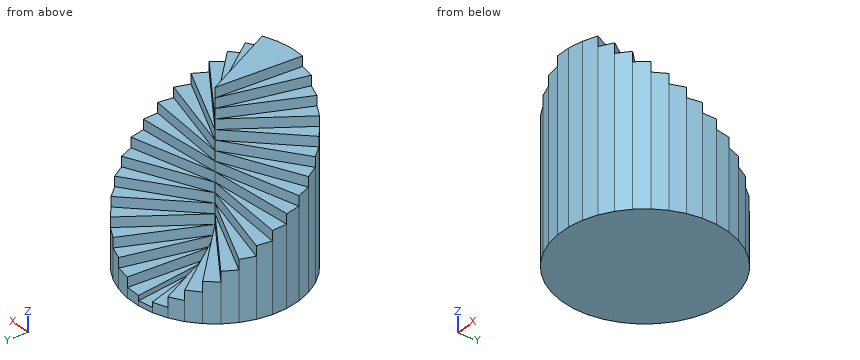
from build123d import *

# Parameters (mm, degrees)
F1_DEPTH  = 2.54
F2_DEPTH  = 5.08
F3_DEPTH  = 7.62
F4_DEPTH  = 10.16
F5_DEPTH  = 12.7
F6_DEPTH  = 15.24
F7_DEPTH  = 17.78
F8_DEPTH  = 20.32
F9_DEPTH  = 22.86
F10_DEPTH = 25.4
F11_DEPTH = 27.94
F12_DEPTH = 30.48
F13_DEPTH = 33.02
F14_DEPTH = 35.56
F15_DEPTH = 38.1
F16_DEPTH = 40.64
F17_DEPTH = 43.18
F18_DEPTH = 43.18
F19_DEPTH = 43.18
F20_DEPTH = 40.64
F21_DEPTH = 38.1
F22_DEPTH = 35.56
F23_DEPTH = 33.02
F24_DEPTH = 30.48
F25_DEPTH = 27.94
F26_DEPTH = 25.4
F27_DEPTH = 22.86
F28_DEPTH = 20.32
F29_DEPTH = 17.78
F30_DEPTH = 15.24
F31_DEPTH = 12.7
F32_DEPTH = 10.16
F33_DEPTH = 7.62
F34_DEPTH = 5.08
F35_DEPTH = 2.54
F36_DEPTH = 1.27


with BuildPart() as f1:
    # F0 (on Top) → F1 (new body)
    with BuildSketch(Plane.XY):
        Polygon((-1.990034, 21.009007), (0, 0), (1.688375, 21.035399), align=None)
    extrude(amount=F1_DEPTH)

    # F0 (on Top) → F2 (join)
    with BuildSketch(Plane.XY):
        Polygon((1.688375, 21.035399), (0, 0), (5.315483, 20.422641), align=None)
    extrude(amount=F2_DEPTH)

    # F0 (on Top) → F3 (join)
    with BuildSketch(Plane.XY):
        Polygon((5.315483, 20.422641), (0, 0), (8.781084, 19.189351), align=None)
    extrude(amount=F3_DEPTH)

    # F0 (on Top) → F4 (join)
    with BuildSketch(Plane.XY):
        Polygon((8.781084, 19.189351), (0, 0), (11.979875, 17.373003), align=None)
    extrude(amount=F4_DEPTH)

    # F0 (on Top) → F5 (join)
    with BuildSketch(Plane.XY):
        Polygon((0, 0), (14.814664, 15.028784), (11.979875, 17.373003), align=None)
    extrude(amount=F5_DEPTH)

    # F0 (on Top) → F6 (join)
    with BuildSketch(Plane.XY):
        Polygon((0, 0), (17.199317, 12.227924), (14.814664, 15.028784), align=None)
    extrude(amount=F6_DEPTH)

    # F0 (on Top) → F7 (join)
    with BuildSketch(Plane.XY):
        Polygon((19.061377, 9.055524), (17.199317, 12.227924), (0, 0), align=None)
    extrude(amount=F7_DEPTH)

    # F0 (on Top) → F8 (join)
    with BuildSketch(Plane.XY):
        Polygon((20.344267, 5.607977), (19.061377, 9.055524), (0, 0), align=None)
    extrude(amount=F8_DEPTH)

    # F0 (on Top) → F9 (join)
    with BuildSketch(Plane.XY):
        Polygon((20.344267, 5.607977), (0, 0), (21.009007, 1.990034), align=None)
    extrude(amount=F9_DEPTH)

    # F0 (on Top) → F10 (join)
    with BuildSketch(Plane.XY):
        Polygon((21.009007, 1.990034), (0, 0), (21.035399, -1.688375), align=None)
    extrude(amount=F10_DEPTH)

    # F0 (on Top) → F11 (join)
    with BuildSketch(Plane.XY):
        Polygon((21.035399, -1.688375), (0, 0), (20.422641, -5.315483), align=None)
    extrude(amount=F11_DEPTH)

    # F0 (on Top) → F12 (join)
    with BuildSketch(Plane.XY):
        Polygon((20.422641, -5.315483), (0, 0), (19.189351, -8.781084), align=None)
    extrude(amount=F12_DEPTH)

    # F0 (on Top) → F13 (join)
    with BuildSketch(Plane.XY):
        Polygon((19.189351, -8.781084), (0, 0), (17.373003, -11.979875), align=None)
    extrude(amount=F13_DEPTH)

    # F0 (on Top) → F14 (join)
    with BuildSketch(Plane.XY):
        Polygon((17.373003, -11.979875), (0, 0), (15.028784, -14.814664), align=None)
    extrude(amount=F14_DEPTH)

    # F0 (on Top) → F15 (join)
    with BuildSketch(Plane.XY):
        Polygon((15.028784, -14.814664), (0, 0), (12.227924, -17.199317), align=None)
    extrude(amount=F15_DEPTH)

    # F0 (on Top) → F16 (join)
    with BuildSketch(Plane.XY):
        Polygon((12.227924, -17.199317), (0, 0), (9.055524, -19.061377), align=None)
    extrude(amount=F16_DEPTH)

    # F0 (on Top) → F17 (join)
    with BuildSketch(Plane.XY):
        Polygon((9.055524, -19.061377), (0, 0), (5.607977, -20.344267), align=None)
    extrude(amount=F17_DEPTH)

    # F0 (on Top) → F18 (join)
    with BuildSketch(Plane.XY):
        Polygon((5.607977, -20.344267), (0, 0), (1.990034, -21.009007), align=None)
    extrude(amount=F18_DEPTH)

    # F0 (on Top) → F19 (join)
    with BuildSketch(Plane.XY):
        Polygon((1.990034, -21.009007), (0, 0), (-1.688375, -21.035399), align=None)
    extrude(amount=F19_DEPTH)

    # F0 (on Top) → F20 (join)
    with BuildSketch(Plane.XY):
        Polygon((-1.688375, -21.035399), (0, 0), (-5.315483, -20.422641), align=None)
    extrude(amount=F20_DEPTH)

    # F0 (on Top) → F21 (join)
    with BuildSketch(Plane.XY):
        Polygon((-5.315483, -20.422641), (0, 0), (-8.781084, -19.189351), align=None)
    extrude(amount=F21_DEPTH)

    # F0 (on Top) → F22 (join)
    with BuildSketch(Plane.XY):
        Polygon((-8.781084, -19.189351), (0, 0), (-11.979875, -17.373003), align=None)
    extrude(amount=F22_DEPTH)

    # F0 (on Top) → F23 (join)
    with BuildSketch(Plane.XY):
        Polygon((-11.979875, -17.373003), (0, 0), (-14.814664, -15.028784), align=None)
    extrude(amount=F23_DEPTH)

    # F0 (on Top) → F24 (join)
    with BuildSketch(Plane.XY):
        Polygon((-14.814664, -15.028784), (0, 0), (-17.199317, -12.227924), align=None)
    extrude(amount=F24_DEPTH)

    # F0 (on Top) → F25 (join)
    with BuildSketch(Plane.XY):
        Polygon((-17.199317, -12.227924), (0, 0), (-19.061377, -9.055524), align=None)
    extrude(amount=F25_DEPTH)

    # F0 (on Top) → F26 (join)
    with BuildSketch(Plane.XY):
        Polygon((-19.061377, -9.055524), (0, 0), (-20.344267, -5.607977), align=None)
    extrude(amount=F26_DEPTH)

    # F0 (on Top) → F27 (join)
    with BuildSketch(Plane.XY):
        Polygon((-20.344267, -5.607977), (0, 0), (-21.009007, -1.990034), align=None)
    extrude(amount=F27_DEPTH)

    # F0 (on Top) → F28 (join)
    with BuildSketch(Plane.XY):
        Polygon((-21.009007, -1.990034), (0, 0), (-21.035399, 1.688375), align=None)
    extrude(amount=F28_DEPTH)

    # F0 (on Top) → F29 (join)
    with BuildSketch(Plane.XY):
        Polygon((-21.035399, 1.688375), (0, 0), (-20.422641, 5.315483), align=None)
    extrude(amount=F29_DEPTH)

    # F0 (on Top) → F30 (join)
    with BuildSketch(Plane.XY):
        Polygon((-20.422641, 5.315483), (0, 0), (-19.189351, 8.781084), align=None)
    extrude(amount=F30_DEPTH)

    # F0 (on Top) → F31 (join)
    with BuildSketch(Plane.XY):
        Polygon((-19.189351, 8.781084), (0, 0), (-17.373003, 11.979875), align=None)
    extrude(amount=F31_DEPTH)

    # F0 (on Top) → F32 (join)
    with BuildSketch(Plane.XY):
        Polygon((-17.373003, 11.979875), (0, 0), (-15.028784, 14.814664), align=None)
    extrude(amount=F32_DEPTH)

    # F0 (on Top) → F33 (join)
    with BuildSketch(Plane.XY):
        Polygon((-15.028784, 14.814664), (0, 0), (-12.227924, 17.199317), align=None)
    extrude(amount=F33_DEPTH)

    # F0 (on Top) → F34 (join)
    with BuildSketch(Plane.XY):
        Polygon((-12.227924, 17.199317), (0, 0), (-9.055524, 19.061377), align=None)
    extrude(amount=F34_DEPTH)

    # F0 (on Top) → F35 (join)
    with BuildSketch(Plane.XY):
        Polygon((-9.055524, 19.061377), (0, 0), (-5.607977, 20.344267), align=None)
    extrude(amount=F35_DEPTH)

    # F0 (on Top) → F36 (join)
    with BuildSketch(Plane.XY):
        Polygon((-5.607977, 20.344267), (0, 0), (-1.990034, 21.009007), align=None)
    extrude(amount=F36_DEPTH)


solid = f1.part
Input: part model. Units: mm. Frame: model coordinates. Give positions to 0.01 mm unless a question says otherwise; leave off trailing zeros. Write each loop counter-clockwise with the first axis right and the second up, starting at its lowest first coordinate (ties: lowest second). Pieces come first, ordered by that corner, then holes. Notation, with made-up numbers: M 68,81 L 99,81 A7 cw 99,94 Z; hole C 84,82 d5. An arc over 180 degrees is marked long. Write item = value, one per line. Start each with the question number.
1) Cut plane C-C on x = -13.5. Return the cut outline in (y, z), then the cut area to 3 significant figures.
2) First-contact query: pin 1 Ø6 at (y, z) = (-15, 15) entering from -X; pin 2 Ø4.5 at (x, y) = (-6, -8) entering from +Z; pin 3 Ø12 at (y, z) = (-4, 23) entering from +X; pin 4 Ø9.5 at (x, y) = (-10.5, 3.5) entering from +Z. Flat tips, straight axial feed; report the tip coordinate or a pass-through.
3) Cut plane A-A on z = 34.5. Return the cut outline in (x, y).
4) Cut plane B-B on y = -8. Return the cut outline in (x, z), then the cut area to 3 significant figures.
5) Material intervals for line 1 along Z through (x, y) = (-1, 11.5); line 2 along Z through (x, y) = (11, -16); line 3 along Y through (x, z) = (-12, 17), sorted ascending. Write a range as [from, to].
6) Cut plane D-D on z = 24.5. Return the cut outline in (x, y).
Solved:
q1.outline = M -16.12,0 L 16.12,0 L 16.12,7.62 L 13.31,7.62 L 13.31,10.16 L 9.31,10.16 L 9.31,12.7 L 6.18,12.7 L 6.18,15.24 L 3.51,15.24 L 3.51,17.78 L 1.08,17.78 L 1.08,20.32 L -1.28,20.32 L -1.28,22.86 L -3.72,22.86 L -3.72,25.4 L -6.41,25.4 L -6.41,27.94 L -9.6,27.94 L -9.6,30.48 L -13.7,30.48 L -13.7,33.02 L -16.12,33.02 Z
q1.area = 652 mm2
q2.pin_1 = -17.33
q2.pin_2 = 38.1
q2.pin_3 = 21.04
q2.pin_4 = 22.86
q3.outline = M -11.98,-17.37 L -8.78,-19.19 L -5.32,-20.42 L -1.69,-21.04 L 1.99,-21.01 L 5.61,-20.34 L 9.06,-19.06 L 12.23,-17.2 L 15.03,-14.81 L 17.37,-11.98 L 0,0 Z
q4.outline = M -19.45,0 L 19.47,0 L 19.47,30.48 L 17.48,30.48 L 17.48,33.02 L 11.6,33.02 L 11.6,35.56 L 8.12,35.56 L 8.12,38.1 L 5.69,38.1 L 5.69,40.64 L 3.8,40.64 L 3.8,43.18 L -0.64,43.18 L -0.64,40.64 L -2.08,40.64 L -2.08,38.1 L -3.66,38.1 L -3.66,35.56 L -5.52,35.56 L -5.52,33.02 L -7.89,33.02 L -7.89,30.48 L -11.25,30.48 L -11.25,27.94 L -16.84,27.94 L -16.84,25.4 L -19.45,25.4 Z
q4.area = 1,330 mm2
q5.line_1 = [0, 2.54]
q5.line_2 = [0, 40.64]
q5.line_3 = [-17.36, 3.12]
q6.outline = M -20.34,-5.61 L -19.06,-9.06 L -17.2,-12.23 L -14.81,-15.03 L -11.98,-17.37 L -8.78,-19.19 L -5.32,-20.42 L -1.69,-21.04 L 1.99,-21.01 L 5.61,-20.34 L 9.06,-19.06 L 12.23,-17.2 L 15.03,-14.81 L 17.37,-11.98 L 19.19,-8.78 L 20.42,-5.32 L 21.04,-1.69 L 21.01,1.99 L 0,0 Z
